Here's the drawing with two shaded views (mm, measured from the low corner). I have some questions. Give positions to 0.01 mm unless a question says otherwise; leave off trailing zeros. Loops run counter-clockwise (first coordinate to the right, second up) from the corner with the lowest first, then second, coordinate; pieces in that order, holes last. Notation, with made-up numbers: (67.25, 38) -> (95.25, 38) arc R24 ccw to (95.25, 66) -> close; hole circle Ø6 at (85, 21). An arc over 180 degrees is marked (long way). Put each result on its own line as item: value.
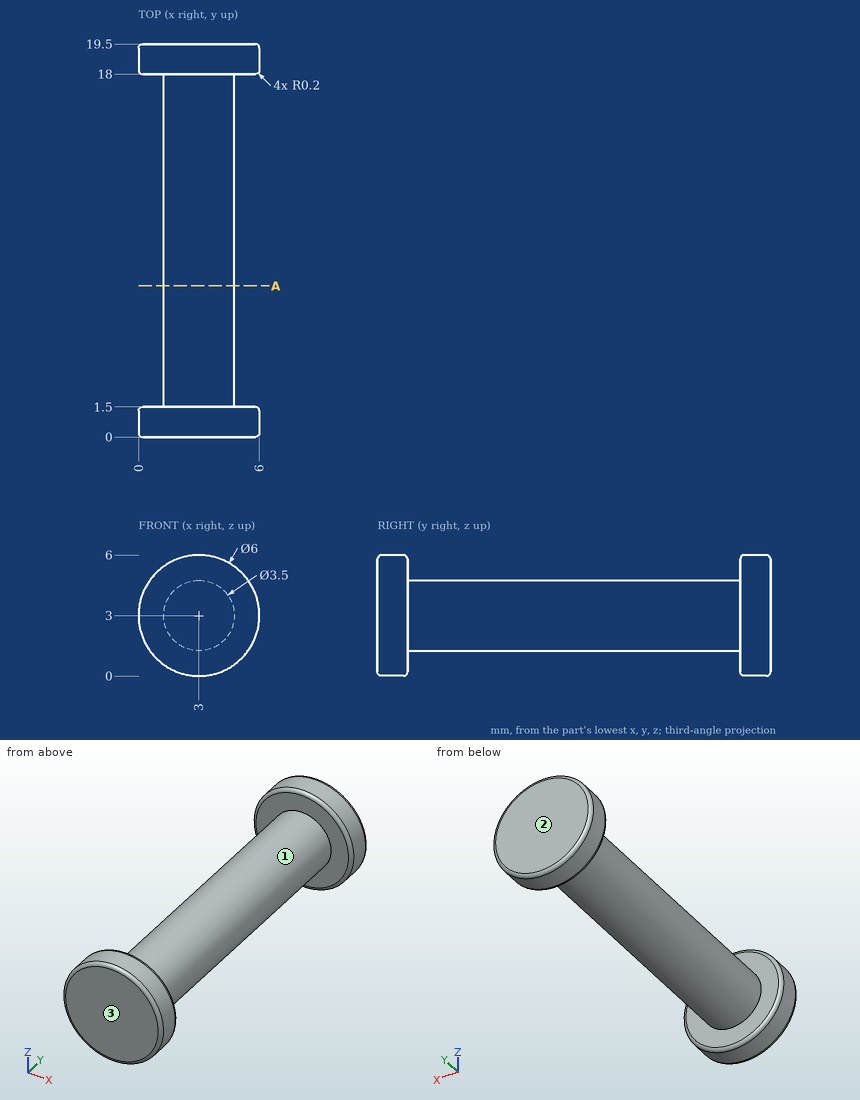
1. Thinking about a two-plate mould opening in Y: for the marked faces 1, 2 and 3, which applies, pulls with the +Y half, pulls with the -Y half, needs draft (parallel to the pull), parting line crosses it, or undercut?
Recorded:
face 1: undercut
face 2: pulls with the +Y half
face 3: pulls with the -Y half
2. If we section it at A-A (y = 7.5): List the corners of the cut face in (x, z) for me.
Recorded:
outline: circle Ø3.5 at (3, 3)
3. I need wall thicknesses on line 1 (Y direction, x = 5, z = 3.5); line 2 (Z direction, x = 2.5, y = 1.25); line 3 (Z direction, x = 4, y = 10.25). Which ranges of each line are inside material? Lowest first, please.
Recorded:
line 1: y = 0 to 1.5, 18 to 19.5
line 2: z = 0.04 to 5.96
line 3: z = 1.56 to 4.44
